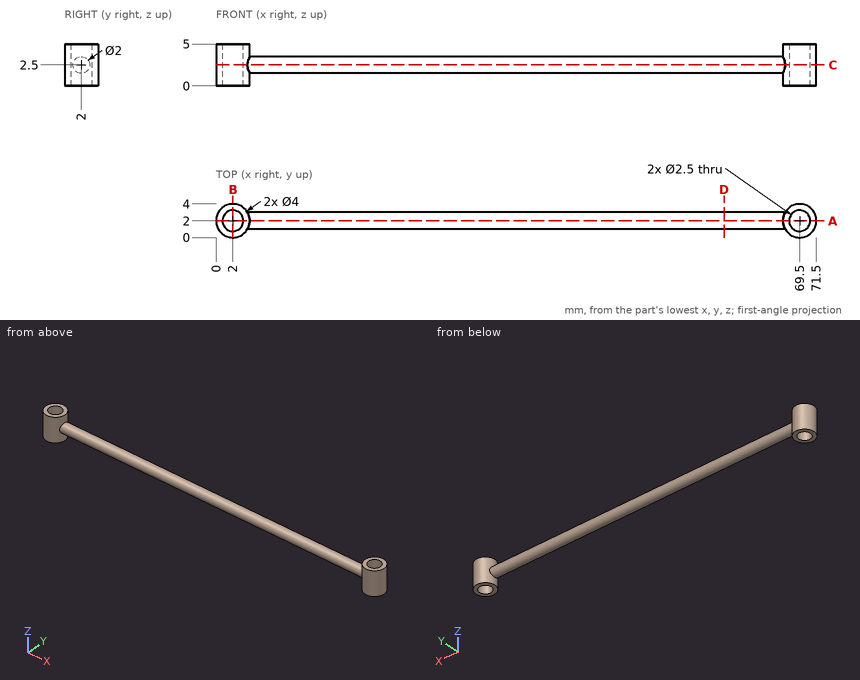
Source: three-view drawing plus pictorial views. Frame: mm from the lowest corner of the part. Round coordinates to 2 decimals unless told otherwise and drop trailing zeros. Write each loop counter-clockwise with the first axis right and the second up, starting at its lowest first coordinate (ties: lowest second). Pieces come first, ordered by that corner, then holes. Notation, with made-up numbers: M 51.5,65 L 98.5,65 A23 cw 98.5,97 Z; hole C -14,-7 d6. An arc over 180 degrees is marked long. Use CSV: the item, a comma, the result in double quotes. Start each with the question number.
Q1. Cut plane D-D on x = 60.5. Output: boundary loops of the cut face in (y, z).
Q2. Cut plane A-A on y = 2. Output: boundary loops of the cut face in (x, z), plus the area to 3 significant figures.
Q3. Cut plane B-B on x = 2. Output: boundary loops of the cut face in (y, z), plus the area to 3 significant figures.
Q4. Cut plane C-C on z = 2.5. Output: boundary loops of the cut face in (x, y).
Q5. First-contact query: P1, Ø1.5, axis at y = 3, z = 4, coming from the -X side; P2, Ø3, axis at x = 49.5, z = 2.5, coming from the +Y side; P3, Ø1.5, axis at y = 3, z = 3.5, coming from the +X side. Flat tips, straight axial feed; report the tip coordinate or a pass-through.
Q6. Line query: line 1 (Y direction, x = 2, z = 2.85); line 2 (X direction, y = 1.7, z = 3.6); line 3 (Z direction, x = 10, y = 2.1). Output: solid intervals per line, ascending. Write a range as from..to.
Results found:
1,outline,"C 2,2.5 d2"
2,outline,"M 0,0 L 0.75,0 L 0.75,5 L 0,5 Z; M 3.25,0 L 4,0 L 4,1.5 L 67.5,1.5 L 67.5,0 L 68.25,0 L 68.25,5 L 67.5,5 L 67.5,3.5 L 4,3.5 L 4,5 L 3.25,5 Z; M 70.75,0 L 71.5,0 L 71.5,5 L 70.75,5 Z"
2,area,"142 mm^2"
3,outline,"M 0,0 L 0.75,0 L 0.75,5 L 0,5 Z; M 3.25,0 L 4,0 L 4,5 L 3.25,5 Z"
3,area,"7.50 mm^2"
4,outline,"M 3.73,1 L 67.77,1 A2 ccw long 67.77,3 L 3.73,3 A2 ccw long Z; hole C 2,2 d2.5; hole C 69.5,2 d2.5"
5,P1,"x = 0.02"
5,P2,"y = 3"
5,P3,"x = 71.48"
6,line 1,"0..0.75, 3.25..4"
6,line 2,"0.02..0.79, 3.21..3.98, 67.52..68.29, 70.71..71.48"
6,line 3,"1.51..3.49"
